```python
from build123d import *

# Parameters (mm, degrees)
F1_DEPTH = 10
F3_R     = 411.0625
F4_DEPTH = 50
F2_W     = 30
F2_H     = 25
F5_DEPTH = 6
F7_DEPTH = 50


with BuildPart() as f1:
    # F0 (on Top) → F1 (new body)
    with BuildSketch(Plane.XY):
        with BuildLine():
            ThreePointArc((17.4375, 11.7018628325), (16.3738601454, 13.1490191245), (15.190457531, 14.5))
            ThreePointArc((15.190457531, 14.5), (0, 21), (-15.190457531, 14.5))
            ThreePointArc((-15.190457531, 14.5), (-16.3738601454, 13.1490191245), (-17.4375, 11.7018628325))
            ThreePointArc((-17.4375, 11.7018628325), (-13.0692952628, 6.561011736), (-11.5, 0))
            ThreePointArc((-11.5, 0), (-13.0692952628, -6.561011736), (-17.4375, -11.7018628325))
            ThreePointArc((-17.4375, -11.7018628325), (-16.3738601454, -13.1490191245), (-15.190457531, -14.5))
            ThreePointArc((-15.190457531, -14.5), (0, -21), (15.190457531, -14.5))
            ThreePointArc((15.190457531, -14.5), (16.3738601454, -13.1490191245), (17.4375, -11.7018628325))
            ThreePointArc((17.4375, -11.7018628325), (11.5, 0), (17.4375, 11.7018628325))
        make_face()
        with BuildLine():
            Line((26, 14.5), (15.190457531, 14.5))
            ThreePointArc((15.190457531, 14.5), (16.3738601454, 13.1490191245), (17.4375, 11.7018628325))
            ThreePointArc((17.4375, 11.7018628325), (21.4959468848, 13.7827248952), (26, 14.5))
        make_face()
        with BuildLine():
            ThreePointArc((-17.4375, 11.7018628325), (-16.3738601454, 13.1490191245), (-15.190457531, 14.5))
            Line((-15.190457531, 14.5), (-26, 14.5))
            ThreePointArc((-26, 14.5), (-21.4959468848, 13.7827248952), (-17.4375, 11.7018628325))
        make_face()
        with BuildLine():
            ThreePointArc((26, 14.5), (21.4959468848, 13.7827248952), (17.4375, 11.7018628325))
            ThreePointArc((17.4375, 11.7018628325), (20.089642854, 6.1160649114), (21, 0))
            ThreePointArc((21, 0), (20.089642854, -6.1160649114), (17.4375, -11.7018628325))
            ThreePointArc((17.4375, -11.7018628325), (21.4959468848, -13.7827248952), (26, -14.5))
            ThreePointArc((26, -14.5), (36.2530483272, -10.2530483272), (40.5, 0))
            ThreePointArc((40.5, 0), (36.2530483272, 10.2530483272), (26, 14.5))
        make_face()
        with BuildLine():
            ThreePointArc((-17.4375, -11.7018628325), (-21, 0), (-17.4375, 11.7018628325))
            ThreePointArc((-17.4375, 11.7018628325), (-21.4959468848, 13.7827248952), (-26, 14.5))
            ThreePointArc((-26, 14.5), (-40.5, 0), (-26, -14.5))
            ThreePointArc((-26, -14.5), (-21.4959468848, -13.7827248952), (-17.4375, -11.7018628325))
        make_face()
        with BuildLine():
            ThreePointArc((26, -14.5), (21.4959468848, -13.7827248952), (17.4375, -11.7018628325))
            ThreePointArc((17.4375, -11.7018628325), (16.3738601454, -13.1490191245), (15.190457531, -14.5))
            Line((15.190457531, -14.5), (26, -14.5))
        make_face()
        with BuildLine():
            ThreePointArc((-15.190457531, -14.5), (-16.3738601454, -13.1490191245), (-17.4375, -11.7018628325))
            ThreePointArc((-17.4375, -11.7018628325), (-21.4959468848, -13.7827248952), (-26, -14.5))
            Line((-26, -14.5), (-15.190457531, -14.5))
        make_face()
        with BuildLine():
            ThreePointArc((-11.5, 0), (-13.0692952628, 6.561011736), (-17.4375, 11.7018628325))
            ThreePointArc((-17.4375, 11.7018628325), (-21, 0), (-17.4375, -11.7018628325))
            ThreePointArc((-17.4375, -11.7018628325), (-13.0692952628, -6.561011736), (-11.5, 0))
        make_face()
        with BuildLine():
            ThreePointArc((21, 0), (20.089642854, 6.1160649114), (17.4375, 11.7018628325))
            ThreePointArc((17.4375, 11.7018628325), (11.5, 0), (17.4375, -11.7018628325))
            ThreePointArc((17.4375, -11.7018628325), (20.089642854, -6.1160649114), (21, 0))
        make_face()
    extrude(amount=F1_DEPTH)

    # F3 (on Front) → F4 (cut, symmetric)
    with BuildSketch(Plane.XZ):
        with Locations((0, -409.0625)):
            Circle(F3_R)
    extrude(amount=F4_DEPTH, both=True, mode=Mode.SUBTRACT)

    # F2 (on face) → F5 (cut)
    with BuildSketch(Plane.XY.offset(10)):
        Rectangle(F2_W, F2_H)
    extrude(amount=-F5_DEPTH, mode=Mode.SUBTRACT)

    # F6 (on Front) → F7 (cut, symmetric)
    with BuildSketch(Plane.XZ):
        with BuildLine():
            ThreePointArc((-40.5, 8), (0, 10), (40.5, 8))
            Line((40.5, 8), (40.5, 38))
            Line((40.5, 38), (-40.5, 38))
            Line((-40.5, 38), (-40.5, 8))
        make_face()
    extrude(amount=F7_DEPTH, both=True, mode=Mode.SUBTRACT)


solid = f1.part
```
For this review, take the finished solid that the model builds, in its own axes (mm). A direction names the side the tool comes from. Round coordinates to 2 decimals unless told otherwise and drop trailing zeros. Order: outer loops, then holes, each group sorted by start corner. A loop starts at its lowest first (then second) coordinate and runs counter-clockwise, first axis right, second up. Notation, with made-up numbers: (83, -7) -> (97, -7) arc R27 ccw to (97, 15) -> close; hole circle Ø11 at (1.5, 54.5). An arc over 180 degrees is marked (long way). Use a Markdown table: item, result.
Item 1: Take a section at C-C (x = 4.5). State the section outline as (y, z) points.
Resolved:
| item | result |
|---|---|
| outline | (-20.51, 1.98) -> (20.51, 1.98) -> (20.51, 9.98) -> (12.5, 9.98) -> (12.5, 4) -> (-12.5, 4) -> (-12.5, 9.98) -> (-20.51, 9.98) -> close |
Item 2: Machinability: for faces 1 (the flat face through (-21, -14.5, 5)), 2 (the flat face through (21, -14.5, 5)), 3 (the flat face through (0, 12.5, 7)), which of the approach directions +Z, -Z, +X, -X, +Y, -Y give a long, thin tool a straight path to every point of the face, cutting with its end or side? Answer none if there is none.
Resolved:
| item | result |
|---|---|
| face 1 | +Z, -Z, -X, -Y |
| face 2 | +Z, -Z, +X, -Y |
| face 3 | +Z |
Item 3: Draft analysis for pull direction Y (two halves, no side actions). For faces 4 (the cylindrical face through (1, 0, 2)), 5 (the flat face through (-15, 0, 7)), 6 (the flat face through (21, 14.5, 5)), state which applies: +Y half, -Y half, draft (parallel to the pull), parting line (faces both ways), or undercut.
Resolved:
| item | result |
|---|---|
| face 4 | draft |
| face 5 | undercut |
| face 6 | +Y half |
Item 4: Take a section at A-A (z = 7). State the section outline as (x, y) points, plus the area to 3 significant figures.
Resolved:
| item | result |
|---|---|
| outline | (-26, -14.5) -> (-15.19, -14.5) arc R21 ccw to (15.19, -14.5) -> (26, -14.5) arc R14.5 ccw to (26, 14.5) -> (15.19, 14.5) arc R21 ccw to (-15.19, 14.5) -> (-26, 14.5) arc R14.5 ccw to start; hole (-15, -12.5) -> (15, -12.5) -> (15, 12.5) -> (-15, 12.5) -> close |
| area | 1,690 mm² |
Item 5: Take a section at B-B (y = 6). State the section outline as (x, z) points (1 decimal).
Resolved:
| item | result |
|---|---|
| outline | (-39.2, 0.1) arc R411.1 cw to (39.2, 0.1) -> (39.2, 8.1) arc R411.1 ccw to (15, 9.7) -> (15, 4) -> (-15, 4) -> (-15, 9.7) arc R411.1 ccw to (-39.2, 8.1) -> close |
Item 6: Take a section at D-D (x = -17). State the section outline as (y, z) points.
Resolved:
| item | result |
|---|---|
| outline | (-14.5, 1.65) -> (14.5, 1.65) -> (14.5, 9.65) -> (-14.5, 9.65) -> close |
Item 7: For pin 1 (2 mm diameter, centred on x = -22.5, z = 2, fed in from -Y); pin 2 (1 mm diameter, centred on x = 24, y = -9, fed in from -Z); pin 3 (5 mm diameter, centred on x = -5.5, z = 7.5, fed in from -Y), all flat-tipped, find the tip position at first contact; note any pin that passes through.
Resolved:
| item | result |
|---|---|
| pin 1 | stops at y = -14.5 |
| pin 2 | stops at z = 1.27 |
| pin 3 | stops at y = -20.78 |
Item 8: For line 1 along Z through (x, y) = (0, -15); line 2 along X through (y, z) = (-11.5, 7); line 3 along Y through (x, z) = (10.5, 6), list the stretches that pass through material, from the lowest coordinate up. Write a range as [from, to].
Resolved:
| item | result |
|---|---|
| line 1 | z = [2, 10] |
| line 2 | x = [-34.83, -15], [15, 34.83] |
| line 3 | y = [-18.19, -12.5], [12.5, 18.19] |
